CAD build for the part. Positions are in the model's coordinates, mm. Face numbers are marked on the shaded views. A direction names the side the tool comes from. Round coordinates to 2 decimals unless told otherwise and drop trailing zeros. Write each loop counter-clockwise with the first axis right and the second up, starting at its lowest first coordinate (ties: lowest second). Pieces come first, ordered by that corner, then holes. Notation, with made-up numbers: (-17.75, 70) - (29.25, 70) arc R12 ccw to (29.25, 88) - close; hole circle Ø4 at (68, 68.5). An arc over 180 degrees is marked (long way). Use one line per item in the form item = value. Start each with the question number.
Item 1: Band-saw the part on C-C, the plane x = 26. List the corners of the cut face in (y, z), and give its area (3 significant figures).
Item 2: Band-saw the part on A-A, the plane z = 0. List the corners of the cut face in (x, y), and give its area (3 significant figures).
Item 3: Pin check, flat tips, straight feed: pin 1 (3.5 mm diameter, centred on x = 50, z = 0, fed in from +Y); pin 2 (1 mm diameter, centred on x = 1, y = -2, fed in from +Z); pin 3 (4 mm diameter, centred on x = -50, z = 0, fed in from -Y); pin 4 (1 mm diameter, centred on y = -1.5, z = 1, fed in from -X). Stop position of each tip, or through.
Item 4: Tool access for the marked faces 1, 2 and 3: list every direction of +Z, -Z, +X, -X, +Y, -Y with a clear straight run to the whole face (end or side of a thin tool).
Item 5: Band-saw the part on B-B, the plane z = -6.75. List the corners of the cut face in (x, y), and give its area (3 significant figures).
Item 6: Drill centre lines: L1, parallel to Z at x = 50, y = -1.6; L2, parallel to Y at x = -25, z = 7; L3, parallel to Y at x = 32, z = 4.25. Where is each one in solid material? Low to high.
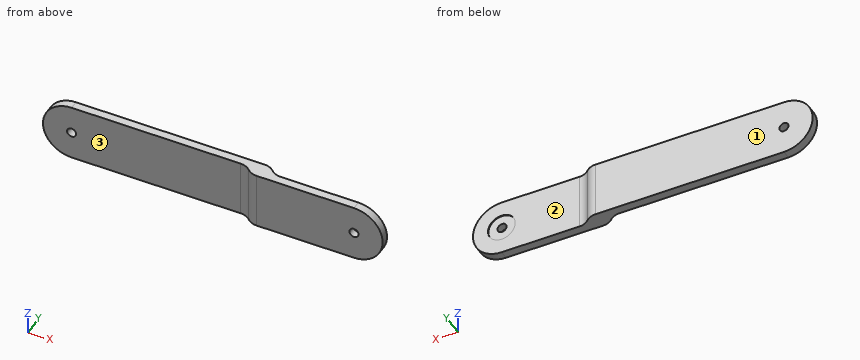
Autodesk Inventor part; units mm, degrees
ref_plane "YZ Plane" through (0, 0, 0) normal (1, 0, 0) x (0, 1, 0)
ref_plane "XZ Plane" through (0, 0, 0) normal (0, 1, 0) x (-1, 0, 0)
ref_plane "XY Plane" through (0, 0, 0) normal (0, 0, 1) x (1, 0, 0)
sketch "Sketch1" plane through (0, 0, 0) normal (0, 1, 0) x (-1, 0, 0)
  line L0 (-50, 10) -> (-18.2962, 10)
  line L1 (-50, -10) -> (-18.2962, -10)
  arc A0 (50, -10) -> (50, 10) centre (50, 0) ccw
  arc A1 (-50, 10) -> (-50, -10) centre (-50, 0) ccw
  circle A2 centre (50, 0) radius 1.6
  line L2 (0, 0) -> (0, -27.365) construction
  line L3 (0, 0) -> (19.8022, 0) construction
  circle A3 centre (50, 0) radius 4.75
  circle A4 centre (-50, 0) radius 1.6
  circle A5 centre (-50, 0) radius 4.75
  line L4 (-13.5485, -10) -> (-13.5485, 10)
  line L5 (-18.2962, -10) -> (-18.2962, 10)
  line L6 (-18.2962, 10) -> (-13.5485, 10)
  line L7 (-13.5485, 10) -> (50, 10)
  line L8 (-18.2962, -10) -> (-13.5485, -10)
  line L9 (-13.5485, -10) -> (50, -10)
  dimension "d1" = 100
  dimension "d2" = 10
  dimension "d3" = 3.2
  dimension "d4" = 9.5
extrude "Extrusion1" add sketch "Sketch1" against normal blind 3 contours L0 L5 L1 A1 | L6 L4 L8 L5 | A5
extrude "Extrusion2" cut sketch "Sketch1" against normal blind 0.3 contours A3 | A5
extrude "Extrusion3" add sketch "Sketch1" along normal blind 3 contours L6 L4 L8 L5 | L7 A0 L9 L4 | A3
fillet "Fillet1" radius 5 4 edges at (18.2962, 3, 0) (18.2962, 0, 0) (13.5485, 0, 0) (13.5485, -3, 0)
properties part number "ramie3"
Determined:
q1.outline = (-3, -10) - (0, -10) - (0, 10) - (-3, 10) - close
q1.area = 60.0 mm²
q2.outline = (-60, 0) - (-51.6, 0) - (-51.6, 3) - (-60, 3) - close; (-48.4, 0) - (8.97, 0) arc R5 cw to (12.54, -1.5) arc R5 ccw to (16.11, -3) - (48.4, -3) - (48.4, -0.3) - (45.25, -0.3) - (45.25, 0) - (22.88, 0) arc R5 cw to (19.31, 1.5) arc R5 ccw to (15.74, 3) - (-48.4, 3) - close; (51.6, -3) - (60, -3) - (60, 0) - (54.75, 0) - (54.75, -0.3) - (51.6, -0.3) - close
q2.area = 359 mm²
q3.pin_1 = -0.3
q3.pin_2 = through
q3.pin_3 = 0
q3.pin_4 = 11.97
q4.face_1 = +Z, -Z, +X, -X, +Y
q4.face_2 = +Z, -Z, +X, +Y
q4.face_3 = +Z, -Z, -X, -Y
q5.outline = (-57.38, 0) - (8.97, 0) arc R5 cw to (12.54, -1.5) arc R5 ccw to (16.11, -3) - (57.38, -3) - (57.38, 0) - (22.88, 0) arc R5 cw to (19.31, 1.5) arc R5 ccw to (15.74, 3) - (-57.38, 3) - close
q5.area = 365 mm²
q6.L1 = -10 to -1.6, 1.6 to 10
q6.L2 = 0 to 3
q6.L3 = -3 to 0
